Autodesk Inventor part; units mm, degrees
ref_plane "YZ Plane" through (0, 0, 0) normal (1, 0, 0) x (0, 1, 0)
ref_plane "XZ Plane" through (0, 0, 0) normal (0, 1, 0) x (-1, 0, 0)
ref_plane "XY Plane" through (0, 0, 0) normal (0, 0, 1) x (1, 0, 0)
sketch "Sketch1" plane through (0, 0, 0) normal (0, 0, 1) x (1, 0, 0)
  line L0 (-23, 42) -> (177, 42)
  line L1 (177, 0) -> (-23, 0)
  line L2 (-63, 0) -> (217, 0)
  line L3 (-23, 42) -> (-23, 32)
  line L4 (-23, 32) -> (-17, 32)
  line L5 (-17, 32) -> (-17, 10)
  line L6 (-17, 10) -> (-23, 10)
  line L7 (-23, 10) -> (-23, 0)
  line L8 (177, 42) -> (177, 32)
  line L9 (177, 32) -> (171, 32)
  line L10 (171, 32) -> (171, 10)
  line L11 (171, 10) -> (177, 10)
  line L12 (177, 10) -> (177, 0)
  circle A0 centre (156, 21) radius 3.5
  circle A1 centre (5, 21) radius 3.5
  point P0 (0, 0)
  point P1 (0, 0)
  dimension "d31" = 200
  dimension "d35" = 6
  dimension "d36" = 10
  dimension "d37" = 10
  dimension "d38" = 23
  dimension "d39" = 10
  dimension "d40" = 10
  dimension "d41" = 6
  dimension "d42" = 7
  dimension "d43" = 15
  dimension "d44" = 21
  dimension "d45" = 42
  dimension "d46" = 10
  dimension "d47" = 7
  dimension "d48" = 21
  dimension "d49" = 28
extrude "Extrusion3" add sketch "Sketch1" along normal blind 6
equation "\"d37\" = d36"
equation "\"d39\" = d36"
equation "\"d40\" = d39"
equation "\"d41\" = d35"
equation "\"d47\" = d42"
equation "\"d48\" = d44"
properties part number "Tope riel motor 2"
The listing builds one solid part. Answer for the finished solid, in the listing's coordinates (mm). A direction names the side the tool comes from. Coordinates: 2 decimals unless noted, no trailing zeros. Loops run counter-clockwise (first coordinate to the right, second up) from the corner with the lowest first, then second, coordinate; pieces in that order, holes last. Notation, with made-up numbers: (47.5, 71.5) -> (100.5, 71.5) arc R29 cw to (100.5, 93.5) -> close; hole circle Ø5 at (56, 64.25). An arc over 180 degrees is marked (long way). Return JSON: item names as keys, results as strings. Group by question number.
(1) Find the intervals of material crossed by probe 1 along X at (y, z) = (20, 5.75); probe 2 along Y at (x, z) = (156, 3.7); probe 3 along X at (y, z) = (12, 1.4), in increasing order. Write a range as from..to.
(2) Given pin 1 Ø5.5 at (x, y) = (5, 21) entering from +Z; pin 2 Ø3 at (x, z) = (136, 5.5) entering from -Y, each flat-ended and moving along its own axis, determine where each tip first touches the part or whether it passes through.
(3) Determine the mould class of faces 1 (the flat face through (174, 10, 3)), 2 (the flat face through (76, 42, 3)), 3 (the flat face through (-23, 5, 3)), 4 (the flat face through (78, 0, 3)) for opening direction Y: released by +Y, released by -Y, zero draft, split by the parting line, or undercut.
(4) A cutting plane is placed at B-B on x = 5. Write down the section's boundary in (y, z), and give its area (3 significant figures).
(5) A cutting plane is placed at C-C on z = 4.45. Write down the section's boundary in (x, y), and give its area (3 significant figures).
(6) A cutting plane is placed at A-A on y = 21. Write down the section's boundary in (x, z), and give its area (3 significant figures).
(7) A cutting plane is placed at D-D on y = 12. Write down the section's boundary in (x, z).
(8) Which of the six approach directions +Z, -Z, +X, -X, +Y, -Y give full straight-line access (tool end or side, diameter ignored) to faces 5 (the flat face through (-23, 37, 3)), 6 (the flat face through (-17, 21, 3)), 7 (the flat face through (174, 32, 3))?
The answers:
{
 "1": {"probe 1": "x = -17..1.65, 8.35..152.65, 159.35..171", "probe 2": "y = 0..17.5, 24.5..42", "probe 3": "x = -17..171"},
 "2": {"pin 1": "passes through", "pin 2": "stops at y = 0"},
 "3": {"face 1": "undercut", "face 2": "released by +Y", "face 3": "zero draft", "face 4": "released by -Y"},
 "4": {"outline": "(0, 0) -> (17.5, 0) -> (17.5, 6) -> (0, 6) -> close; (24.5, 0) -> (42, 0) -> (42, 6) -> (24.5, 6) -> close", "area": "210 mm^2"},
 "5": {"outline": "(-23, 0) -> (177, 0) -> (177, 10) -> (171, 10) -> (171, 32) -> (177, 32) -> (177, 42) -> (-23, 42) -> (-23, 32) -> (-17, 32) -> (-17, 10) -> (-23, 10) -> close; hole circle Ø7 at (5, 21); hole circle Ø7 at (156, 21)", "area": "8,060 mm^2"},
 "6": {"outline": "(-17, 0) -> (1.5, 0) -> (1.5, 6) -> (-17, 6) -> close; (8.5, 0) -> (152.5, 0) -> (152.5, 6) -> (8.5, 6) -> close; (159.5, 0) -> (171, 0) -> (171, 6) -> (159.5, 6) -> close", "area": "1,040 mm^2"},
 "7": {"outline": "(-17, 0) -> (171, 0) -> (171, 6) -> (-17, 6) -> close"},
 "8": {"face 5": "+Z, -Z, -X, +Y, -Y", "face 6": "+Z, -Z, -X", "face 7": "+Z, -Z, +X"}
}
